Autodesk Inventor part; units mm, degrees
ref_plane "YZ Plane" through (0, 0, 0) normal (1, 0, 0) x (0, 1, 0)
ref_plane "XY Plane" through (0, 0, 0) normal (0, 0, 1) x (1, 0, 0)
sketch "スケッチ1" plane through (0, 0, 0) normal (0, 0, 1) x (1, 0, 0)
  arc A0 (0, 100) -> (0, -100) centre (0, 0) ccw
  line L0 (0, 100) -> (0, -100)
  dimension "d0" = 200
revolve "回転1" add sketch "スケッチ1" angle 360 about axis through (0, 100, 0) along (0, -1, 0)
sketch "スケッチ2" plane through (0, 0, 0) normal (0, 1, 0) x (-1, 0, 0)
  line L0 (140.6562, -148.6683) -> (-138.1636, -148.6683)
  line L1 (-138.1636, -148.6683) -> (-138.1636, -69.972)
  line L2 (-138.1636, -69.972) -> (140.6562, -69.972)
  line L3 (140.6562, -69.972) -> (140.6562, -148.6683)
  point P0 (0, 0)
extrude "押し出し1" cut sketch "スケッチ2" along normal mid plane 200
sketch "スケッチ3" plane through (0, 0, 0) normal (0, 1, 0) x (-1, 0, 0)
  circle A0 centre (0, 0) radius 25
  dimension "d4" = 50
extrude "押し出し2" cut sketch "スケッチ3" along normal mid plane 200
properties part number "HeadP"
Read the model definition and answer for the solid it produces. Units are mm, in the model's axes. Coordinates: 2 decimals unless noted, no trailing zeros. Order: outer loops, then holes, each group sorted by start corner. A loop starts at its lowest first (then second) coordinate and runs counter-clockwise, first axis right, second up. Notation, with made-up numbers: (38, -40) - (68, -40) arc R22 ccw to (68, -6) - close; hole circle Ø2 at (71.25, 78.25). An arc over 180 degrees is marked (long way). Use one line per item in the form item = value.
(1) Given pin 1 Ø12 at (y, z) = (77.5, 22.5) entering from -X; pin 2 Ø10 at (y, z) = (49, -30) entering from +X; pin 3 Ø5 at (x, z) = (4, 76) entering from +Y, each flat-ended and moving along its own axis, determine where each tip first touches the part or whether it passes through.
Computed values:
pin_1 = -66.48
pin_2 = 85.14
pin_3 = 67.69
(2) Section C-C, the plane y = 41 is taken. Give the vertices of the cut face in (x, z), then the cut area to 3 significant figures.
Computed values:
outline = (-58.51, -69.97) - (58.51, -69.97) arc R91.21 ccw (long way) to start; hole circle Ø50 at (0, 0)
area = 22,500 mm²
(3) Section B-B, the plane z = 0 is taken. Give the vertices of the cut face in (x, y).
Computed values:
outline = (-25, -96.82) - (-25, 96.82) arc R100 ccw to start; (25, -96.82) arc R100 ccw to (25, 96.82) - close
(4) Section A-A, the plane x = 0 is taken. Give the vertices of the cut face in (y, z), then the cut area to 3 significant figures.
Computed values:
outline = (-96.82, -25) arc R100 ccw to (-71.44, -69.97) - (71.44, -69.97) arc R100 ccw to (96.82, -25) - close; (-96.82, 25) - (96.82, 25) arc R100 ccw to start
area = 18,600 mm²
(5) Section D-D, the plane x = 28 is taken. Give the vertices of the cut face in (y, z), then the cut area to 3 significant figures.
Computed values:
outline = (-65.73, -69.97) - (65.73, -69.97) arc R96 ccw (long way) to start
area = 26,600 mm²
(6) Straight lines are drawn through the part: L1, parallel to X at y = 73, z = -7.5; L2, parallel to X at y = 20, z = 0; L3, parallel to Z at x = -1, y = -21.5. For each, find the intervals that lie inside material, in ascending order.
Computed values:
L1 = -67.93 to -23.85, 23.85 to 67.93
L2 = -97.98 to -25, 25 to 97.98
L3 = -69.97 to -24.98, 24.98 to 97.66
